For this review, take the finished solid that the model builds, in its own axes (mm). Round coordinates to 2 decimals unless told otherwise and drop trailing zeros. Order: outer loops, then holes, each group sorted by start corner. A loop starts at its lowest first (then second) coordinate and runs counter-clockwise, first axis right, second up. Notation, with made-up numbers: M -15.5,71.25 L -7.5,71.25 A13 ccw -7.5,76.25 Z; hole C 14,-31 d3. An arc over 180 degrees is marked long. Put each result on its own line as item: value.
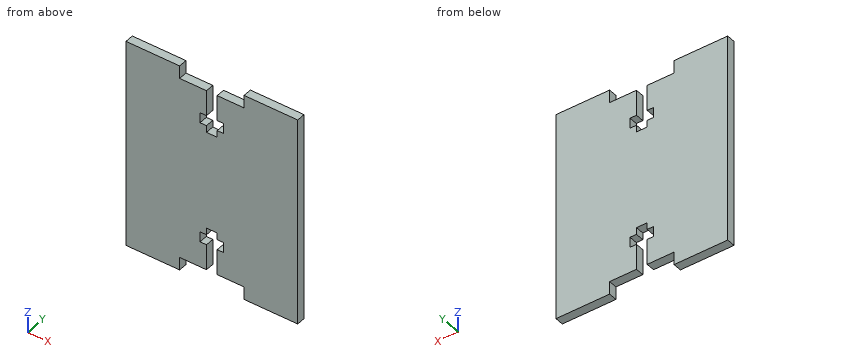
from build123d import *

# Parameters (mm, degrees)
SCHIZZO1_W                   = 40
SCHIZZO1_H                   = 49
ESTRUSIONE_ESTRUSIONE2_DEPTH = 2
SCHIZZO2_W                   = 15
SCHIZZO2_H                   = 3
TAGLIO_ESTRUSIONE1_DEPTH     = 3
TAGLIO_ESTRUSIONE3_DEPTH     = 3


with BuildPart() as part:
    # Schizzo1 → Estrusione-Estrusione2 (new body)
    with BuildSketch(Plane(origin=(0, 0, 0), x_dir=(1, 0, 0), z_dir=(0, 1, 0))):
        with Locations((-34.56494914, -3.781075862)):
            Rectangle(SCHIZZO1_W, SCHIZZO1_H)
    extrude(amount=-ESTRUSIONE_ESTRUSIONE2_DEPTH)

    # Schizzo2 → Taglio-Estrusione1 (cut, through all)
    with BuildSketch(Plane(origin=(0, 0, 0), x_dir=(1, 0, 0), z_dir=(0, 1, 0))):
        with Locations((-34.56494914, -26.781075862)):
            Rectangle(SCHIZZO2_W, SCHIZZO2_H)
        with Locations((-34.56494914, 19.218924138)):
            Rectangle(SCHIZZO2_W, SCHIZZO2_H)
    extrude(amount=-TAGLIO_ESTRUSIONE1_DEPTH, mode=Mode.SUBTRACT)

    # Schizzo3 → Taglio-Estrusione3 (cut, through all)
    with BuildSketch(Plane(origin=(0, 0, 0), x_dir=(1, 0, 0), z_dir=(0, 1, 0))):
        Polygon((-35.81494914, -25.281075862), (-33.31494914, -25.281075862), (-33.31494914, -19.281075862), (-31.81494914, -19.281075862), (-31.81494914, -16.881075862), (-33.31494914, -16.881075862), (-33.31494914, -15.281075862), (-35.81494914, -15.281075862), (-35.81494914, -16.881075862), (-37.31494914, -16.881075862), (-37.31494914, -19.281075862), (-35.81494914, -19.281075862), align=None)
        Polygon((-35.81494914, 7.718924138), (-33.31494914, 7.718924138), (-33.31494914, 9.318924138), (-31.81494914, 9.318924138), (-31.81494914, 11.718924138), (-33.31494914, 11.718924138), (-33.31494914, 17.718924138), (-35.81494914, 17.718924138), (-35.81494914, 11.718924138), (-37.31494914, 11.718924138), (-37.31494914, 9.318924138), (-35.81494914, 9.318924138), align=None)
    extrude(amount=-TAGLIO_ESTRUSIONE3_DEPTH, mode=Mode.SUBTRACT)


solid = part.part
(1) Add section C-C on z = -12.5. Give the boundary of the cut face in (x, y).
A:
outline: M -54.56,-2 L -35.81,-2 L -35.81,0 L -54.56,0 Z; M -33.31,-2 L -14.56,-2 L -14.56,0 L -33.31,0 Z
(2) Add section B-B on x = -40.5. Give the boundary of the cut face in (y, z).
A:
outline: M -2,-17.72 L 0,-17.72 L 0,25.28 L -2,25.28 Z
(3) To check wall thickness, follow L1, parallel to Z at x = -36, y = -1.75; L2, parallel to X at y = -1.1, z = 18.5; L3, parallel to X at y = -0.45, z = 26. State the ranges of each line that lie inside material, in increasing order.
A:
L1: z = -17.72 to -11.72, -9.32 to 16.88, 19.28 to 25.28
L2: x = -54.56 to -37.31, -31.81 to -14.56
L3: x = -54.56 to -42.06, -27.06 to -14.56
(4) Add section A-A on z = 17.5. Give the boundary of the cut face in (x, y), then the cut area to 3 significant figures.
A:
outline: M -54.56,-2 L -37.31,-2 L -37.31,0 L -54.56,0 Z; M -31.81,-2 L -14.56,-2 L -14.56,0 L -31.81,0 Z
area: 69.0 mm2
(5) Insertion check: pin 1 Ø0.8 at (x, y) = (-32.5, -0.5) entering from +Z; pin 2 Ø1 at (x, y) = (-34.5, -0.5) entering from +Z; pin 3 Ø0.6 at (x, y) = (-39.5, -0.5) entering from -Z. Each pin has a flat end and moves straight along its axis. Give the tip position at first contact, or say it passes through.
A:
pin 1: stops at z = 25.28
pin 2: stops at z = 15.28
pin 3: stops at z = -17.72
